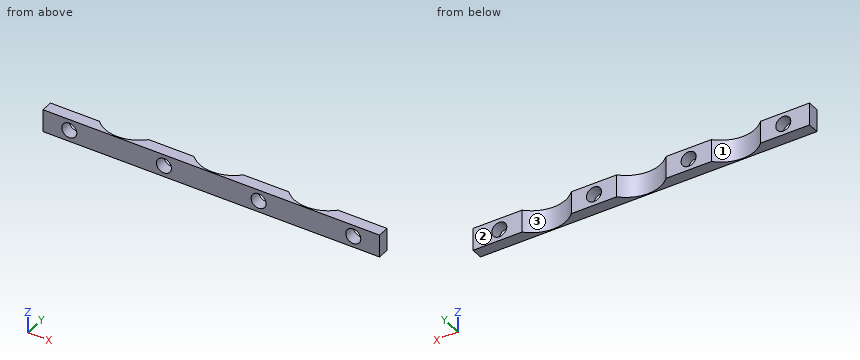
from build123d import *

# Parameters (mm, degrees)
BOSS_EXTRUDE1_DEPTH = 4.3
SKETCH2_R           = 1.425
CUT_EXTRUDE1_DEPTH  = 33.362478273


with BuildPart() as part:
    # Sketch1 → Boss-Extrude1 (new body)
    with BuildSketch(Plane.XY):
        with BuildLine():
            Line((-13.312338898, -10.5), (-4.69041576, -10.5))
            ThreePointArc((-4.69041576, -10.5), (0, -12.5), (4.69041576, -10.5))
            Line((4.69041576, -10.5), (13.312338898, -10.5))
            ThreePointArc((13.312338898, -10.5), (18.002754658, -12.5), (22.693170418, -10.5))
            Line((22.693170418, -10.5), (32, -10.5))
            Line((32, -10.5), (32, -12.7))
            Line((32, -12.7), (-32, -12.7))
            Line((-32, -12.7), (-32, -10.5))
            Line((-32, -10.5), (-22.693170418, -10.5))
            ThreePointArc((-22.693170418, -10.5), (-18.002754658, -12.5), (-13.312338898, -10.5))
        make_face()
    extrude(amount=BOSS_EXTRUDE1_DEPTH)

    # Sketch2 → Cut-Extrude1 (cut, through all)
    with BuildSketch(Plane(origin=(0, -10.5, 0), x_dir=(1, 0, 0), z_dir=(0, 1, 0))):
        with Locations(Location((-9, -2.15, 0), (0, 0, 180))):
            Circle(SKETCH2_R)
        with Locations(Location((9, -2.15, 0), (0, 0, 180))):
            Circle(SKETCH2_R)
        with Locations(Location((-27, -2.15, 0), (0, 0, 180))):
            Circle(SKETCH2_R)
        with Locations(Location((27, -2.15, 0), (0, 0, 180))):
            Circle(SKETCH2_R)
    extrude(amount=-CUT_EXTRUDE1_DEPTH, mode=Mode.SUBTRACT)


solid = part.part
Could you check a few things on this model? Use its own coordinates, in mm. Face numbers are marked on the shaded views. Give positions to 0.01 mm unless a question says otherwise; leave off trailing zeros. Loops run counter-clockwise (first coordinate to the right, second up) from the corner with the lowest first, then second, coordinate; pieces in that order, holes last. Notation, with made-up numbers: (5, 55.25) -> (47, 55.25) arc R30 cw to (47, 93.25) -> close; hole circle Ø8 at (11, -16). An arc over 180 degrees is marked (long way). Return JSON: item names as keys, results as strings.
Item 1: I need wall thicknesses on L1, parallel to Z at x = 27, y = -12.2 (3 decimals); L2, parallel to X at y = -11.45, z = 3.9 (1 decimal); L3, parallel to X at y = -11.35, z = 0.65. Which ranges of each line are inside material? Lowest first, please. Write a range as from..to.
Geometry results:
{"L1": "z = 0..0.725, 3.575..4.3", "L2": "x = -32..-21.5, -14.5..-3.5, 3.5..14.5, 21.5..32", "L3": "x = -32..-21.69, -14.31..-3.69, 3.69..14.31, 21.69..32"}
Item 2: We'd pull the mould along X, two halves only. Please class the marked faces 1, 2 and 3: +X half, -X half, draft (parallel to the pull), parting line (faces both ways), or undercut.
Geometry results:
{"face 1": "undercut", "face 2": "draft", "face 3": "undercut"}
Item 3: If we section it at D-D on x = -18: List the corners of the cut face in (y, z) for me.
Geometry results:
{"outline": "(-12.7, 0) -> (-12.5, 0) -> (-12.5, 4.3) -> (-12.7, 4.3) -> close"}
Item 4: If we section it at A-A on y = -12.15: List the corners of the cut face in (x, z) for me (3 decimals), plus the area to 3 significant figures.
Geometry results:
{"outline": "(-32, 0) -> (-20.107, 0) -> (-20.107, 4.3) -> (-32, 4.3) -> close; (-15.899, 0) -> (-2.104, 0) -> (-2.104, 4.3) -> (-15.899, 4.3) -> close; (2.104, 0) -> (15.899, 0) -> (15.899, 4.3) -> (2.104, 4.3) -> close; (20.107, 0) -> (32, 0) -> (32, 4.3) -> (20.107, 4.3) -> close; hole circle Ø2.85 at (-27, 2.15); hole circle Ø2.85 at (-9, 2.15); hole circle Ø2.85 at (9, 2.15); hole circle Ø2.85 at (27, 2.15)", "area": "195 mm²"}
Item 5: I'm going to push flat-ended pins straight in: pin 1 (1.7 mm diameter, centred on x = 27, z = 2.15, fed in from -Y); pin 2 (2 mm diameter, centred on x = -21.5, z = 2.5, fed in from +Y). Where does each tip first touch, or does it pass through?
Geometry results:
{"pin 1": "passes through", "pin 2": "stops at y = -10.69"}
Item 6: If we section it at B-B on z = 2.15: List the corners of the cut face in (x, y) for me (3 decimals), plus the area to 3 significant figures.
Geometry results:
{"outline": "(-32, -12.7) -> (-28.425, -12.7) -> (-28.425, -10.5) -> (-32, -10.5) -> close; (-25.575, -12.7) -> (-10.425, -12.7) -> (-10.425, -10.5) -> (-13.312, -10.5) arc R6.5 cw to (-22.693, -10.5) -> (-25.575, -10.5) -> close; (-7.575, -12.7) -> (7.575, -12.7) -> (7.575, -10.5) -> (4.69, -10.5) arc R6.5 cw to (-4.69, -10.5) -> (-7.575, -10.5) -> close; (10.425, -12.7) -> (25.575, -12.7) -> (25.575, -10.5) -> (22.693, -10.5) arc R6.5 cw to (13.312, -10.5) -> (10.425, -10.5) -> close; (28.425, -12.7) -> (32, -12.7) -> (32, -10.5) -> (28.425, -10.5) -> close", "area": "76.9 mm²"}
Item 7: If we section it at C-C on x = -9: List the corners of the cut face in (y, z) for me (3 decimals).
Geometry results:
{"outline": "(-12.7, 0) -> (-10.5, 0) -> (-10.5, 0.725) -> (-12.7, 0.725) -> close; (-12.7, 3.575) -> (-10.5, 3.575) -> (-10.5, 4.3) -> (-12.7, 4.3) -> close"}
